from build123d import *

# Parameters (mm, degrees)
SKETCH1_R           = 12.25
BOSS_EXTRUDE1_DEPTH = 11
SKETCH2_R           = 16
BOSS_EXTRUDE2_DEPTH = 2
SKETCH4_R           = 10
BOSS_EXTRUDE4_DEPTH = 1
SKETCH5_R           = 8.5
BOSS_EXTRUDE5_DEPTH = 12
SKETCH6_R           = 6
CUT_EXTRUDE1_DEPTH  = 35.467375879
CHAMFER1_SIZE       = 1
BOSS_EXTRUDE6_START = 2
SKETCH3_R           = 16
BOSS_EXTRUDE6_DEPTH = 2


with BuildPart() as part:
    # Sketch1 → Boss-Extrude1 (new body)
    with BuildSketch(Plane.XY):
        Circle(SKETCH1_R)
    extrude(amount=BOSS_EXTRUDE1_DEPTH)

    # Sketch2 → Boss-Extrude2 (add)
    with BuildSketch(Plane(origin=(0, 0, 0), x_dir=(-1, 0, 0), z_dir=(0, 0, -1))):
        Circle(SKETCH2_R)
    extrude(amount=BOSS_EXTRUDE2_DEPTH)

    # Sketch4 → Boss-Extrude4 (add)
    with BuildSketch(Plane(origin=(0, 0, -2), x_dir=(-1, 0, 0), z_dir=(0, 0, -1))):
        Circle(SKETCH4_R)
    extrude(amount=BOSS_EXTRUDE4_DEPTH)

    # Sketch5 → Boss-Extrude5 (add)
    with BuildSketch(Plane(origin=(0, 0, -3), x_dir=(-1, 0, 0), z_dir=(0, 0, -1))):
        Circle(SKETCH5_R)
    extrude(amount=BOSS_EXTRUDE5_DEPTH)

    # Sketch6 → Cut-Extrude1 (cut, through all)
    with BuildSketch(Plane(origin=(0, 0, -15), x_dir=(-1, 0, 0), z_dir=(0, 0, -1))):
        Circle(SKETCH6_R)
    extrude(amount=-CUT_EXTRUDE1_DEPTH, mode=Mode.SUBTRACT)

    # Chamfer1
    chamfer1_edges = [part.edges().sort_by_distance(p)[0] for p in [
        (6, 0, -15),
    ]]
    chamfer(chamfer1_edges, length=CHAMFER1_SIZE)

    # Sketch3 → Boss-Extrude6 (add)
    with BuildSketch(Plane.XY.offset(11).offset(BOSS_EXTRUDE6_START)):
        with Locations(Location((0, 0, 0), (0, 0, 180))):
            Circle(SKETCH3_R)
    extrude(amount=-BOSS_EXTRUDE6_DEPTH)


solid = part.part
Build history of the part. All positions in model axes, mm. A direction names the side the tool comes from. Give positions to 0.01 mm unless a question says otherwise; leave off trailing zeros. Order: outer loops, then holes, each group sorted by start corner. A loop starts at its lowest first (then second) coordinate and runs counter-clockwise, first axis right, second up. Notation, with made-up numbers: M 28.5,16.25 L 50.5,16.25 A12 ccw 50.5,27.25 Z; hole C 11.5,53.5 d7. An arc over 180 degrees is marked long. Use one line per item in the form item = value.
1) Tool access for faces 5 (the face through (-2, 7, -15)), 6 (the face through (2.17, -9.76, -2.49)), 7 (the face through (4, 12, 11)): list every direction of +Z, -Z, +X, -X, +Y, -Y with a clear straight run to the whole face (end or side of a thin tool).
Calculated:
face_5 = -Z, +X, -X, +Y, -Y
face_6 = -Z
face_7 = none
2) Probe probe 1 along Z at (x, y) = (13, 3); probe 2 along Y at (x, z) = (0, -5); probe 3 along Y at (x, z) = (0, 1). List the from-to ranges inside material, lowest first.
Calculated:
probe_1 = -2 to 0, 11 to 13
probe_2 = -8.5 to -6, 6 to 8.5
probe_3 = -12.25 to -6, 6 to 12.25
3) Saw through at C-C (z = -3.5). Give the cut face in (x, y), plus the area to 3 significant figures.
Calculated:
outline = C 0,0 d17; hole C 0,0 d12
area = 114 mm2
4) Drop flat-ended pins along their axis: pin 1 (4 mm diameter, centred on x = -7.5, y = 4.5, fed in from -Z); pin 2 (4 mm diameter, centred on x = 3, z = 1.5, fed in from +Y); pin 3 (3.5 mm diameter, centred on x = -0.5, y = 2, fed in from -Z); pin 4 (2 mm diameter, centred on x = -3, y = 10.5, fed in from -Z). Give the stop position or say it passes through.
Calculated:
pin_1 = -15
pin_2 = 15.91
pin_3 = 11
pin_4 = -3
5) Two-plate mould, pull along Z, no slides. Class faces 1 (the face through (3.47, 15.62, 12.01)), 2 (the face through (4, -12, 0)), 3 (the face through (6.586, 10.329, 5.423)), 4 (the face through (-10.4, 0.2, -2)): released by +Z, released by -Z, zero draft, split by the parting line, or undercut.
Calculated:
face_1 = zero draft
face_2 = undercut
face_3 = undercut
face_4 = released by -Z
6) Saw through at D-D (x = 13). Give the cut face in (y, z), plus the area to 3 significant figures.
Calculated:
outline = M -9.33,-2 L 9.33,-2 L 9.33,0 L -9.33,0 Z; M -9.33,11 L 9.33,11 L 9.33,13 L -9.33,13 Z
area = 74.6 mm2
7) Saw through at A-A (y = 0). Give the cut face in (x, z), plus the area to 4 significant figures.
Calculated:
outline = M -16,-2 L -10,-2 L -10,-3 L -8.5,-3 L -8.5,-15 L -7,-15 L -6,-14 L -6,11 L 6,11 L 6,-14 L 7,-15 L 8.5,-15 L 8.5,-3 L 10,-3 L 10,-2 L 16,-2 L 16,0 L 12.25,0 L 12.25,11 L 16,11 L 16,13 L -16,13 L -16,11 L -12.25,11 L -12.25,0 L -16,0 Z
area = 308.5 mm2
